CAD build for the part. Positions are in the model's coordinates, mm. Coordinates: 2 decimals unless noted, no trailing zeros. Order: outer loops, then holes, each group sorted by start corner. A loop starts at its lowest first (then second) coordinate and runs counter-clockwise, first axis right, second up. Notation, with made-up numbers: M 71,86.5 L 92,86.5 A25 cw 92,109.5 Z; hole C 30.25,-9 d3. An arc over 180 degrees is marked long. Write item = value, one per line. Start each with the question number.
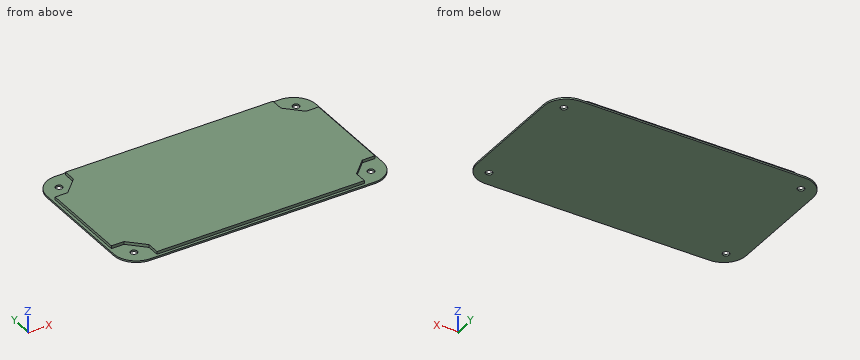
```python
from build123d import *

# Parameters (mm, degrees)
BOSS_EXTRUDE1_DEPTH     = 1.5
CUT_EXTRUDE1_DEPTH      = 138.689868908
CUT_EXTRUDE1_DEPTH_BACK = 138.689868908
SKETCH2_R               = 3
BOSS_EXTRUDE2_DEPTH     = 2.5


with BuildPart() as part:
    # Sketch1 → Boss-Extrude1 (new body)
    with BuildSketch(Plane.XY):
        with BuildLine():
            Line((-100, -67.5), (100, -67.5))
            ThreePointArc((100, -67.5), (114.142135624, -61.642135624), (120, -47.5))
            Line((120, -47.5), (120, 47.5))
            ThreePointArc((120, 47.5), (114.142135624, 61.642135624), (100, 67.5))
            Line((100, 67.5), (-100, 67.5))
            ThreePointArc((-100, 67.5), (-114.142135624, 61.642135624), (-120, 47.5))
            Line((-120, 47.5), (-120, -47.5))
            ThreePointArc((-120, -47.5), (-114.142135624, -61.642135624), (-100, -67.5))
        make_face()
    extrude(amount=BOSS_EXTRUDE1_DEPTH)

    # Sketch2 → Cut-Extrude1 (cut, two sides: drawn at the far end of the back side and taken through both)
    with BuildSketch(Plane.XY.offset(1.5).offset(-CUT_EXTRUDE1_DEPTH_BACK)):
        with Locations((105.710599836, 53.210599836)):
            Circle(SKETCH2_R)
        with Locations((105.710599836, -53.210599836)):
            Circle(SKETCH2_R)
        with Locations((-105.710599836, -53.210599836)):
            Circle(SKETCH2_R)
        with Locations((-105.710599836, 53.210599836)):
            Circle(SKETCH2_R)
    extrude(amount=CUT_EXTRUDE1_DEPTH + CUT_EXTRUDE1_DEPTH_BACK, mode=Mode.SUBTRACT)

    # Sketch2_3 → Boss-Extrude2 (add)
    with BuildSketch(Plane.XY.offset(1.5)):
        Polygon((-106.25, -40), (-92.5, -53.75), (-92.5, -65), (92.5, -65), (92.5, -53.75), (106.25, -40), (117.5, -40), (117.5, 40), (106.25, 40), (92.5, 53.75), (92.5, 65), (-92.5, 65), (-92.5, 53.75), (-106.25, 40), (-117.5, 40), (-117.5, -40), align=None)
    extrude(amount=BOSS_EXTRUDE2_DEPTH)


solid = part.part
```
1. Slice it at A-A (x = 47). Write the cut outline in (y, z).
2. Probe L1, parallel to Y at x = 90, z = 2; L2, parallel to X at y = -32, z = 2.8; L3, parallel to X at y = -59.5, z = 1.9. List the from-to ranges inside material, lowest first.
3. Flat gauge pins, fed straight in: pin 1 (8 mm diameter, centred on x = -63.5, y = 50.5, fed in from -Z); pin 2 (8 mm diameter, centred on x = 105.71, y = 53.21, fed in from +Z); pin 3 (1.2 mm diameter, centred on x = 45, z = 3.5, fed in from -Y); pin 4 (2 mm diameter, centred on x = -110.5, z = 2, fed in from +Y). Where does each tip first touch, or does it go through?
4. Slice it at B-B (z = 2.9). Write the cut outline in (x, y), plus the area to 3 significant figures.
Calculated:
q1.outline = M -67.5,0 L 67.5,0 L 67.5,1.5 L 65,1.5 L 65,4 L -65,4 L -65,1.5 L -67.5,1.5 Z
q2.L1 = -65 to 65
q2.L2 = -117.5 to 117.5
q2.L3 = -92.5 to 92.5
q3.pin_1 = 0
q3.pin_2 = 1.5
q3.pin_3 = -65
q3.pin_4 = 65.03
q4.outline = M -117.5,-40 L -106.25,-40 L -92.5,-53.75 L -92.5,-65 L 92.5,-65 L 92.5,-53.75 L 106.25,-40 L 117.5,-40 L 117.5,40 L 106.25,40 L 92.5,53.75 L 92.5,65 L -92.5,65 L -92.5,53.75 L -106.25,40 L -117.5,40 Z
q4.area = 28,400 mm²
